Autodesk Inventor part; units mm, degrees
ref_plane "Work Plane1" through (0, 0, 0) normal (0, 0, 1) x (1, 0, 0)
ref_plane "YZ Plane" through (0, 0, 0) normal (1, 0, 0) x (0, 1, 0)
ref_plane "XZ Plane" through (0, 0, 0) normal (0, 1, 0) x (-1, 0, 0)
ref_plane "Work Plane1" through (0, 0, 0) normal (0, 0, 1) x (1, 0, 0)
sketch "Sketch1" plane through (0, 0, 0) normal (0, 0, 1) x (1, 0, 0)
  line L0 (-0.508, 0) -> (-0.508, -400)
  line L1 (-5.768, 0) -> (-5.768, -400)
  circle A0 centre (-3.138, -50.8) radius 2.63
  line L2 (-13.138, 0) -> (-13.138, -400)
  circle A1 centre (-3.138, -50.8) radius 7.3925 construction
  line L3 (-3.138, -58.1925) -> (-15.838, -58.1925)
  line L4 (-15.838, -58.1925) -> (-15.838, -43.4075)
  line L5 (-15.838, -43.4075) -> (-3.138, -43.4075)
  arc A2 (-3.138, -58.1925) -> (-3.138, -43.4075) centre (-3.138, -50.8) ccw
  point P0 (0, 0)
  dimension "d0" = 5.26
  dimension "d1" = 10
  dimension "d2" = 4.7625
  dimension "d3" = 12.7
  dimension "d4" = 50.8
extrude "Extrusion1" add sketch "Sketch1" along normal blind 8.2625 contours A2 L0 | L0 A0 L1 L5 A2 | L0 A2 L3 L1 A0 | L1 L3 L2 L5 | L2 L3 L4 L5
sketch "Sketch2" plane through (0, 0, 8.2625) normal (0, 0, 1) x (1, 0, 0)
  line L0 (-15.838, -43.4075) -> (-15.838, -58.1925)
  line L1 (-15.838, -58.1925) -> (-3.138, -58.1925)
  arc A0 (-3.138, -58.1925) -> (-3.138, -43.4075) centre (-3.138, -50.8) ccw
  line L2 (-3.138, -43.4075) -> (-15.838, -43.4075)
  circle A1 centre (-3.138, -50.8) radius 2.63
  line L3 (-3.138, -43.4075) -> (-15.838, -43.4075)
  line L4 (-12.663, -43.4075) -> (-12.663, -58.1925)
  point P0 (0, 0)
  dimension "d7" = 3.175
extrude "Extrusion2" add sketch "Sketch2" along normal blind 12.7 contours L2 L4 L1 L0
sketch "Sketch3" plane through (-15.838, -43.4075, 0) normal (0, 1, 0) x (1, 0, 0)
  circle A0 centre (9.525, -14.6125) radius 6.35 construction
  line L0 (12.7, -8.2625) -> (3.175, -8.2625)
  line L1 (3.175, -8.2625) -> (3.175, -20.9625)
  line L2 (3.175, -20.9625) -> (9.525, -20.9625)
  arc A1 (9.525, -8.2625) -> (9.525, -20.9625) centre (9.525, -14.6125) ccw
  point P0 (15.838, 0)
  point P1 (3.175, -14.6125)
  dimension "d10" = 12.7
extrude "Extrusion3" add sketch "Sketch3" against normal up to surface (14.785 mm away)
fillet "Fillet1" radius 0.0247 1 edges at (-6.313, -50.8, 20.9625)
chamfer "Chamfer1" distance 0.7937 angle 45 2 edges at (-15.838, -50.8, 0) (-15.838, -50.8, 20.9625)
sketch "Sketch4" plane through (-3.138, -43.4075, 8.2625) normal (0, 1, 0) x (1, 0, 0)
  arc A0 (-3.175, 0) -> (-3.9641, -12.6508) centre (-3.175, -6.35) ccw
  arc A1 (-3.9641, -12.6508) -> (-2.6216, -12.6758) centre (-3.175, -6.35) ccw
  arc A2 (-3.9672, -12.7) -> (-3.9641, -12.6508) centre (-3.9672, -12.6753) ccw
  line L0 (-3.175, -6.35) -> (-2.6216, -12.6758) construction
  line L1 (-3.175, -6.35) -> (-3.175, -12.7) construction
  line L2 (-2.6216, -12.6758) -> (-2.6216, -14.2875)
  line L3 (-2.6216, -14.2875) -> (-12.7, -14.2875)
  line L4 (-11.9062, -12.7) -> (-12.7, -11.9062)
  line L5 (-12.7, -14.2875) -> (-12.7, -11.9062)
  line L6 (-11.9062, -12.7) -> (-3.9672, -12.7)
  point P0 (3.138, 8.2625)
  point P1 (-3.9425, -12.6768)
  dimension "d18" = 5
  dimension "d19" = 1.5875
extrude "Extrusion4" add sketch "Sketch4" against normal up to surface (14.785 mm away)
fillet "Fillet2" radius 0.3969 1 edges at (-5.7596, -50.8, 20.9383)
chamfer "Chamfer2" distance 0.3969 angle 45 2 edges at (-5.7596, -50.8, 22.55) (-15.838, -50.8, 22.55)
sketch "Sketch5" plane through (0, 0, 8.2625) normal (0, 0, 1) x (1, 0, 0)
  circle A0 centre (-3.138, -50.8) radius 2.63
  circle A1 centre (-3.138, -50.8) radius 5
  point P0 (0, 0)
  dimension "d26" = 10
extrude "Extrusion5" cut sketch "Sketch5" along normal mid plane 10
properties part number "CNC-029-WireConduitHolder"
Read the model definition and answer for the solid it produces. Units are mm, in the model's axes. Round coordinates to 2 decimals unless told otherwise and drop trailing zeros. Write each loop counter-clockwise with the first axis right and the second up, starting at its lowest first coordinate (ties: lowest second). Pieces come first, ordered by that corner, then holes. Notation, with made-up numbers: (44, 47.25) - (87, 47.25) arc R14 ccw to (87, 58.25) - close; hole circle Ø10 at (-32, -3.5). An arc over 180 degrees is marked (long way). One line per question, with ' | ' between items. Start each with the question number.
1. Section C-C (y = -50.8) is taken. Determine the outline of the cut face in (x, z), and give its area (3 significant figures).
2. Section B-B (z = 5.25) is taken. Determine the outline of the cut face in (x, y) (1 decimal), and give its area (3 significant figures).
3. Each of these flat-tipped pins is pushed along its axis until it touches: pin 1 (2 mm diameter, centred on y = -48.5, z = 6.5, fed in from +X); pin 2 (0.9 mm diameter, centred on y = -53, z = 22, fed in from +X); pin 3 (5.5 mm diameter, centred on x = -1, y = -53, fed in from +Z). Where does it stop, or does it pass through?
4. For a pull along X with two mould halves and no side action, classify faces 1 (the face through (-15.838, -51, 12)), 2 (the face through (-8.133, -50.58, 5.933)), 3 (the face through (-1, -53, 3.262)), 4 (the face through (-11, -43.408, 9)) as +X half, -X half, draft (parallel to the pull), parting line (faces both ways), or undercut.
5. Section D-D (x = -2.5) is taken. Determine the outline of the cut face in (y, z), and give its area (3 significant figures).
6. Find the intervals of material crossed by probe 1 along Z at (x, y) = (-6.25, -56); probe 2 along Z at (x, y) = (0.75, -45.25); probe 3 along Z at (x, y) = (0.75, -49.75), in increasing order. Write a range as [from, to].
7. Section A-A (x = -11.75) is taken. Determine the outline of the cut face in (y, z).
Filled in:
1) outline: (-15.84, 0.79) - (-15.04, 0) - (-5.77, 0) - (-5.77, 3.26) - (-8.14, 3.26) - (-8.14, 8.53) arc R6.35 cw to (-7.1, 20.91) arc R6.34 cw to (-6.17, 20.96) arc R0.4 ccw to (-5.76, 21.36) - (-5.76, 22.15) - (-6.16, 22.55) - (-15.44, 22.55) - (-15.84, 22.15) - close; (-0.51, 0) - (4.25, 0) - (4.25, 8.26) - (1.86, 8.26) - (1.86, 3.26) - (-0.51, 3.26) - close | area: 172 mm²
2) outline: (-15.8, -58.2) - (-3.1, -58.2) arc R7.4 ccw to (-3.1, -43.4) - (-15.8, -43.4) - close; hole circle Ø10 at (-3.1, -50.8) | area: 195 mm²
3) pin 1: x = 4.14 | pin 2: x = -5.76 | pin 3: z = 8.26
4) face 1: -X half | face 2: undercut | face 3: undercut | face 4: draft
5) outline: (-58.16, 0) - (-53.35, 0) - (-53.35, 3.26) - (-55.76, 3.26) - (-55.76, 8.26) - (-58.16, 8.26) - close; (-48.25, 0) - (-43.44, 0) - (-43.44, 8.26) - (-45.84, 8.26) - (-45.84, 3.26) - (-48.25, 3.26) - close | area: 55.5 mm²
6) probe 1: [0, 8.26], [20.96, 22.55] | probe 2: [0, 8.26] | probe 3: [0, 3.26]
7) outline: (-58.19, 0) - (-43.41, 0) - (-43.41, 11.33) - (-58.19, 11.33) - close; (-58.19, 17.89) - (-43.41, 17.89) - (-43.41, 22.55) - (-58.19, 22.55) - close
